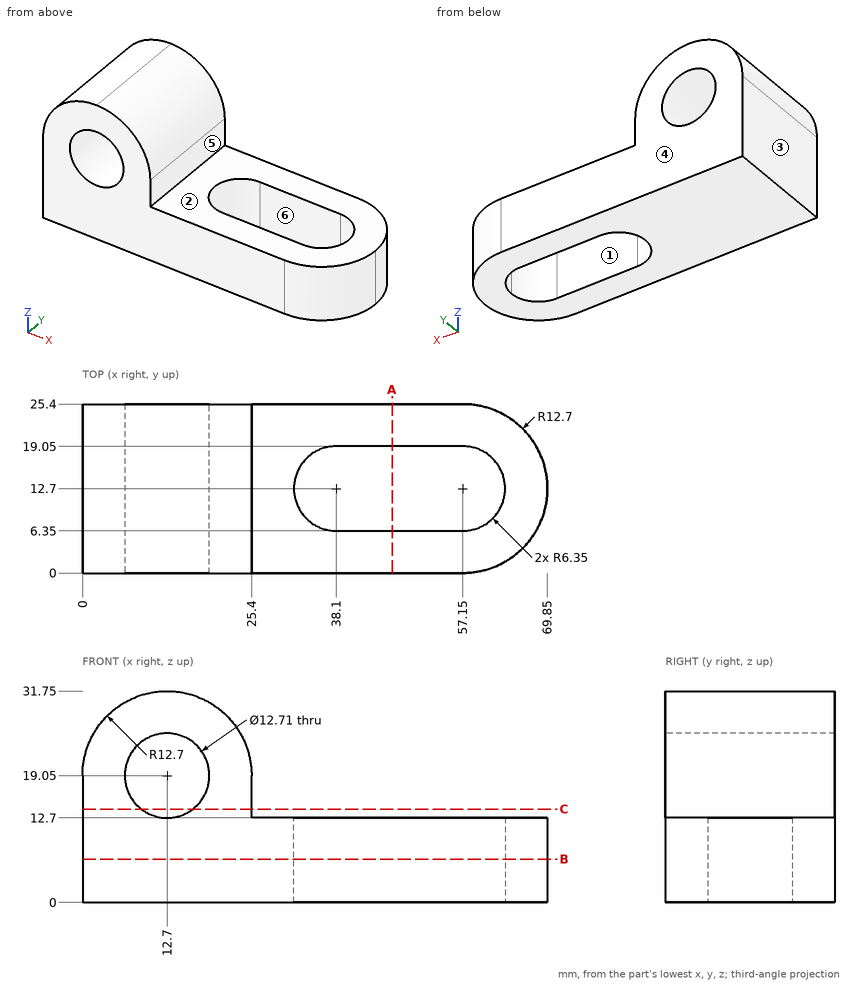
Could you check a few things on this drawing? It's one solid part, dimensions in mm from its lowest x, y, z. A direction names the side the tool comes from. Round coordinates to 2 decimals unless told otherwise and drop trailing zeros. Loops run counter-clockwise (first coordinate to the right, second up) from the corner with the lowest first, then second, coordinate; pieces in that order, holes last. Notation, with made-up numbers: M -28.75,5.5 L -9.75,5.5 A8 cw -9.75,19.5 Z; hole C -20,12.5 d10. An arc over 180 degrees is marked long. Write item = value, one per line. Start each with the question number.
(1) I need wall thicknesses on line 1 along Z through (x, y) = (12.7, 20.75) (3 decimals); line 2 along Y through (x, z) = (39, 11); line 3 along X through (y, z) = (17.25, 24) (1 decimal). Which ranges of each line are inside material? Lowest first, please.
(2) Which directions (+Z, -Z, +X, -X, +Y, -Y) give clear straight access to the entire face, cutting with the end or side of a thin tool? Please do the marked faces 1, 2 and 3.
(3) I'm going to push flat-ended pins straight in: P1, Ø6, axis at x = 10.5, z = 19.5, coming from the -Y side; P2, Ø4, axis at y = 7.5, z = 8, coming from the +X side; P3, Ø12.5, axis at x = 45.5, y = 17, coming from the +Z side; P4, Ø4, axis at y = 10, z = 24, coming from the -X side. Where does each tip first touch, or does it pass through?
(4) Suppose I cut it at B-B on z = 6.5. Write out the boundary of the cut face in (x, y), plus the area to 3 significant figures.
(5) If we mould it in two halves opening along X, with no side actions, what happens to the marked faces 4, 5 and 6? For each: released by +X, released by -X, zero draft, split by the parting line, or undercut.
(6) Suppose I cut it at C-C on z = 14. Write out the boundary of the cut face in (x, y).
(7) Suppose I cut it at A-A on x = 46.5. Write out the boundary of the cut face in (y, z), plus the area to 3 significant figures.
Answer block:
q1.line_1 = 0 to 12.695, 25.405 to 31.75
q1.line_2 = 0 to 6.35, 19.05 to 25.4
q1.line_3 = 1 to 8.7, 16.7 to 24.4
q2.face_1 = +Z, -Z
q2.face_2 = +Z, +X, +Y, -Y
q2.face_3 = +Z, -Z, -X, +Y, -Y
q3.P1 = through
q3.P2 = 69.44
q3.P3 = 12.7
q3.P4 = 0.35
q4.outline = M 0,0 L 57.15,0 A12.7 ccw 57.15,25.4 L 0,25.4 Z; hole M 38.1,6.35 L 57.15,6.35 A6.35 ccw 57.15,19.05 L 38.1,19.05 A6.35 ccw Z
q4.area = 1,340 mm²
q5.face_4 = zero draft
q5.face_5 = released by +X
q5.face_6 = undercut
q6.outline = M 0,0 L 8.84,0 L 8.84,25.4 L 0,25.4 Z; M 16.56,0 L 25.4,0 L 25.4,25.4 L 16.56,25.4 Z
q7.outline = M 0,0 L 6.35,0 L 6.35,12.7 L 0,12.7 Z; M 19.05,0 L 25.4,0 L 25.4,12.7 L 19.05,12.7 Z
q7.area = 161 mm²
